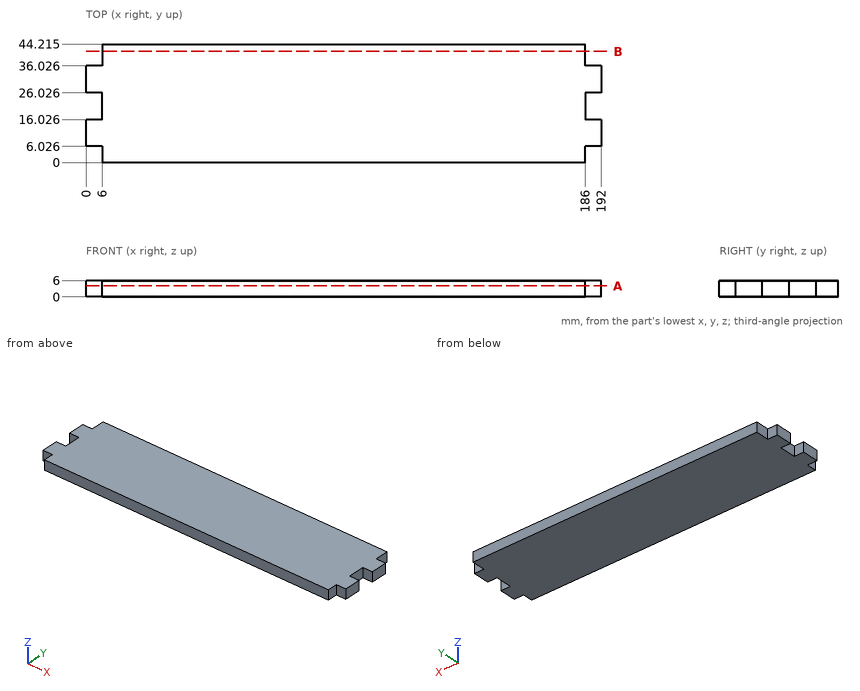
Answer from the drawing. Dimensions are ordinates in mm from the lowest x, y and z of the part. Round coordinates to 2 decimals unless told otherwise and drop trailing zeros. Loops run counter-clockwise (first coordinate to the right, second up) from the corner with the lowest first, then second, coordinate; pieces in that order, holes last. Notation, with made-up numbers: (-29.75, 53) - (-10.75, 53) arc R16 ccw to (-10.75, 63) - close; hole circle Ø5 at (-17.5, 73.25). An arc over 180 degrees is marked (long way). Return JSON: item names as keys, results as strings. Group by question number.
1. Each of these flat-tipped pins is pushed along its axis until it touches: P1, Ø3, axis at y = 3.5, z = 1.5, coming from the +X side; P2, Ø3, axis at x = 188.5, z = 1.5, coming from the -Y side; P3, Ø1.8, axis at x = 190, z = 2.5, coming from the +Y side. Where does it stop, or does it pass through?
2. The part is cut by section B-B on y = 41.5. Determine the outline of the cut face in (x, z).
3. The part is cut by section A-A on z = 4.05. Determine the outline of the cut face in (x, y) (1 decimal).
4. Consider probe 1 along X at (y, z) = (24, 4.1). Determine where the line is inside the solid, lowest interval first.
Resolved:
{
 "1": {"P1": "stops at x = 186", "P2": "stops at y = 6.03", "P3": "stops at y = 36.03"},
 "2": {"outline": "(6, 0) - (186, 0) - (186, 6) - (6, 6) - close"},
 "3": {"outline": "(0, 6) - (6, 6) - (6, 0) - (186, 0) - (186, 6) - (192, 6) - (192, 16) - (186, 16) - (186, 26) - (192, 26) - (192, 36) - (186, 36) - (186, 44.2) - (6, 44.2) - (6, 36) - (0, 36) - (0, 26) - (6, 26) - (6, 16) - (0, 16) - close"},
 "4": {"probe 1": "x = 6 to 186"}
}
